from build123d import *

# Parameters (mm, degrees)
BOSS_EXTRU_1_DEPTH   = 8
D_GAGEMENT_M52_D     = 5.8
D_GAGEMENT_M52_DEPTH = 90
D_GAGEMENT_M52_TIP   = 1.742495795


with BuildPart() as part:
    # Esquisse1 → Boss.-Extru.1 (new body)
    with BuildSketch(Plane.XY):
        with BuildLine():
            Line((-20, 56.568542495), (-73.333333333, 37.712361663))
            ThreePointArc((-73.333333333, 37.712361663), (-100, 0), (-73.333333333, -37.712361663))
            Line((-73.333333333, -37.712361663), (-20, -56.568542495))
            ThreePointArc((-20, -56.568542495), (34.641016151, -48.989794856), (60, 0))
            ThreePointArc((60, 0), (34.641016151, 48.989794856), (-20, 56.568542495))
        make_face()
    extrude(amount=BOSS_EXTRU_1_DEPTH)

    # Dégagement M52
    with Locations(Plane(origin=(15, 0, 8), x_dir=(0, 1, 0), z_dir=(0, 0, 1))):
        with Locations((43.604918173, 41.666666667), (0, -35), (-43.301270189, -10), (43.301270189, -10), (-22.360679775, 95), (22.360679775, 95), (-43.604918173, 41.666666667)):
            Hole(D_GAGEMENT_M52_D / 2, depth=D_GAGEMENT_M52_DEPTH)
            with Locations((0, 0, -(D_GAGEMENT_M52_DEPTH + D_GAGEMENT_M52_TIP / 2))):  # 118° drill point
                Cone(0, D_GAGEMENT_M52_D / 2, D_GAGEMENT_M52_TIP, mode=Mode.SUBTRACT)


solid = part.part
Input: part model. Units: mm. Frame: model coordinates. Give positions to 0.01 mm unless a question says otherwise; leave off trailing zeros. Loops run counter-clockwise (first coordinate to the right, second up) from the corner with the lowest first, then second, coordinate; pieces in that order, holes last. Notation, with made-up numbers: M 34,52.5 L 90,52.5 A32 ccw 90,90.5 Z; hole C -22,57 d5. An arc over 180 degrees is marked long. Use one line per item in the form item = value.
1. Pull-direction query (Y, two-part tool) for faces 1 (the face through (-99.994, 0.689, 3.944)), 2 (the face through (-29.112, 42.046, 3.944)), 3 (the face through (-47.04, -47.01, 3.94)); classes: released by +Y, released by -Y, zero draft, split by the parting line, or undercut.
Numbers:
face_1 = split by the parting line
face_2 = undercut
face_3 = released by -Y
2. Section query C-C, the plane y = 22. Return the cut outline in (x, z).
Numbers:
outline = M -93.41,0 L -82.88,0 L -82.88,8 L -93.41,8 Z; M -77.12,0 L 55.82,0 L 55.82,8 L -77.12,8 Z
3. Section query A-A, the plane x = 25. Return the cut outline in (y, z).
Numbers:
outline = M -54.54,0 L -46.2,0 L -46.2,8 L -54.54,8 Z; M -40.4,0 L 40.4,0 L 40.4,8 L -40.4,8 Z; M 46.2,0 L 54.54,0 L 54.54,8 L 46.2,8 Z
4. Section query B-B, the plane y = -44.5. Return the cut outline in (x, z) (3 decimals).
Numbers:
outline = M -54.135,0 L -29.425,0 L -29.425,8 L -54.135,8 Z; M -23.908,0 L 22.359,0 L 22.359,8 L -23.908,8 Z; M 27.641,0 L 40.246,0 L 40.246,8 L 27.641,8 Z
5. Line query: L1, parallel to Y at x = 25, z = 2.25; L2, parallel to Y at x = -80, z = 4.75; L3, parallel to Y at x = 1.5, z = 6.25. Output: solid intervals per line, ascending.
Numbers:
L1 = -54.54 to -46.2, -40.4 to 40.4, 46.2 to 54.54
L2 = -34.64 to -25.26, -19.46 to 19.46, 25.26 to 34.64
L3 = -59.98 to 59.98
6. First-contact query: pin 1 (4 mm diameter, centred on x = -13, z = 2, fed in from -Y); pin 2 (4 mm diameter, centred on x = -4, z = 6.5, fed in from +Y); pin 3 (1 mm diameter, centred on x = 6.5, z = 1, fed in from -Y). Flat tips, straight axial feed; report the tip coordinate or a pass-through.
Numbers:
pin_1 = -58.98
pin_2 = 59.97
pin_3 = -59.7
7. Section query D-D, the plane z = 6. Return the cut outline in (x, y), and give its area (3 significant figures).
Numbers:
outline = M -73.33,-37.71 L -20,-56.57 A60 ccw long -20,56.57 L -73.33,37.71 A40 ccw Z; hole C -80,-22.36 d5.8; hole C -80,22.36 d5.8; hole C -26.67,-43.6 d5.8; hole C -26.67,43.6 d5.8; hole C 25,-43.3 d5.8; hole C 25,43.3 d5.8; hole C 50,0 d5.8
area = 14,300 mm²
